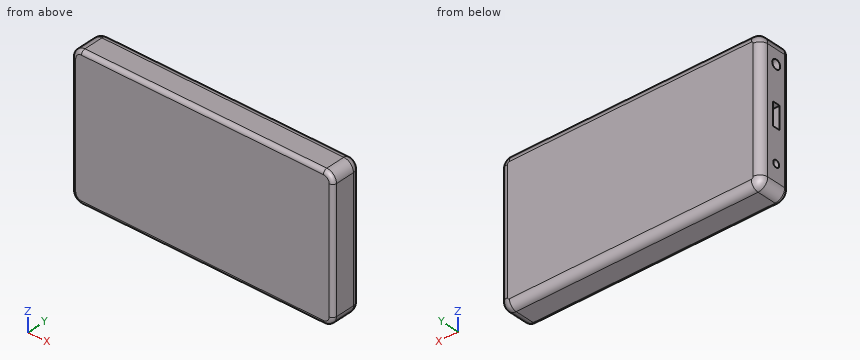
```python
from build123d import *

# Parameters (mm, degrees)
SKETCH1_W           = 270
SKETCH1_H           = 145
BOSS_EXTRUDE1_DEPTH = 32
FILLET1_R           = 8
FILLET2_R           = 10
FILLET3_R           = 4
SKETCH2_R           = 3.521962556
SKETCH2_R_2         = 4.707421484
SKETCH2_W           = 23.153777818
SKETCH2_H           = 8.080231906
CUT_EXTRUDE1_DEPTH  = 33


with BuildPart() as part:
    # Sketch1 → Boss-Extrude1 (new body)
    with BuildSketch(Plane(origin=(0, 0, 0), x_dir=(1, 0, 0), z_dir=(0, 1, 0))):
        Rectangle(SKETCH1_W, SKETCH1_H)
    extrude(amount=BOSS_EXTRUDE1_DEPTH)

    # Fillet1
    fillet1_edges = [part.edges().sort_by_distance(p)[0] for p in [
        (-135, 32, 0),
        (0, 32, 72.5),
        (135, 32, 0),
        (0, 32, -72.5),
    ]]
    fillet(fillet1_edges, radius=FILLET1_R)

    # Fillet2
    # the kernel refuses this fillet: 10 mm, written as the material it takes off along each edge
    with BuildSketch(Plane(origin=(-125, 32, 62.5), x_dir=(-1, 0, 0), z_dir=(0, 0, -1))) as fillet2_piece_1:
        with BuildLine():
            CenterArc((2, -8), 8, 0, 90)
            Line((10, -8), (10, 0))
            Line((10, 0), (2, 0))
        make_face()
    revolve(axis=Axis((-125, 32, 62.5), (0, 1, 0)), revolution_arc=90, mode=Mode.SUBTRACT)
    with BuildSketch(Plane(origin=(-125, 32, -62.5), x_dir=(0, 0, -1), z_dir=(1, 0, 0))) as fillet2_piece_2:
        with BuildLine():
            CenterArc((2, -8), 8, 0, 90)
            Line((10, -8), (10, 0))
            Line((10, 0), (2, 0))
        make_face()
    revolve(axis=Axis((-125, 32, -62.5), (0, 1, 0)), revolution_arc=90, mode=Mode.SUBTRACT)
    with BuildSketch(Plane(origin=(125, 32, 62.5), x_dir=(0, 0, 1), z_dir=(-1, 0, 0))) as fillet2_piece_3:
        with BuildLine():
            CenterArc((2, -8), 8, 0, 90)
            Line((10, -8), (10, 0))
            Line((10, 0), (2, 0))
        make_face()
    revolve(axis=Axis((125, 32, 62.5), (0, 1, 0)), revolution_arc=90, mode=Mode.SUBTRACT)
    with BuildSketch(Plane(origin=(125, 32, -62.5), x_dir=(1, 0, 0), z_dir=(0, 0, 1))) as fillet2_piece_4:
        with BuildLine():
            CenterArc((2, -8), 8, 0, 90)
            Line((10, -8), (10, 0))
            Line((10, 0), (2, 0))
        make_face()
    revolve(axis=Axis((125, 32, -62.5), (0, 1, 0)), revolution_arc=90, mode=Mode.SUBTRACT)
    with BuildSketch(Plane(origin=(135, -25, -72.5), x_dir=(-1, 0, 0), z_dir=(0, 1, 0)), Plane(origin=(135, -25, 72.5), x_dir=(0, 0, -1), z_dir=(0, 1, 0))) as fillet2_piece_5:
        with BuildLine():
            CenterArc((FILLET2_R, FILLET2_R), FILLET2_R, 180, 90)
            Line((0, FILLET2_R), (0, 0))
            Line((0, 0), (FILLET2_R, 0))
        make_face()
    extrude(amount=57, mode=Mode.SUBTRACT)
    with BuildSketch(Plane(origin=(-135, -25, -72.5), x_dir=(1, 0, 0), z_dir=(0, 1, 0)), Plane(origin=(-135, -25, 72.5), x_dir=(0, 0, -1), z_dir=(0, 1, 0))) as fillet2_piece_6:
        with BuildLine():
            CenterArc((FILLET2_R, -FILLET2_R), FILLET2_R, 90, 90)
            Line((0, -FILLET2_R), (0, 0))
            Line((0, 0), (FILLET2_R, 0))
        make_face()
    extrude(amount=57, mode=Mode.SUBTRACT)

    # Fillet3
    fillet3_edges = [part.edges().sort_by_distance(p)[0] for p in [
        (-135, 0, 0),
        (135, 0, 0),
        (0, 0, 72.5),
        (0, 0, -72.5),
        (132.071067812, 0, 69.571067812),
        (132.071067812, 0, -69.571067812),
        (-132.071067812, 0, 69.571067812),
        (-132.071067812, 0, -69.571067812),
    ]]
    fillet(fillet3_edges, radius=FILLET3_R)

    # Sketch2 → Cut-Extrude1 (cut)
    with BuildSketch(Plane.ZY.offset(135)):
        with Locations((-45.200201046, 14)):
            Circle(SKETCH2_R)
        with Locations((48.220259023, 14)):
            Circle(SKETCH2_R_2)
        with Locations((0, 14)):
            Rectangle(SKETCH2_W, SKETCH2_H)
    extrude(amount=-CUT_EXTRUDE1_DEPTH, mode=Mode.SUBTRACT)


solid = part.part
```
Here's how the part is built. I have some questions about the finished solid (model axes, mm). Coordinates: 2 decimals unless noted, no trailing zeros. Order: outer loops, then holes, each group sorted by start corner. A loop starts at its lowest first (then second) coordinate and runs counter-clockwise, first axis right, second up. Notation, with made-up numbers: (59, 24.5) - (103, 24.5) arc R19 ccw to (103, 46.5) - close; hole circle Ø8 at (54.5, 10). An arc over 180 degrees is marked (long way). One line per question, with ' | ' between items. Start each with the question number.
1. If we section it at A-A (y = 14): Write out the boundary of the cut face in (x, z), and give its area (3 significant figures).
2. Please list where these lines run through material, in increasing order: line 1 along Z through (x, y) = (-116, 13); line 2 along X through (y, z) = (25, 8); line 3 along X through (y, z) = (24.5, -44). Write a range as [from, to].
3. I'm going to push a flat-ended pin straight in: pin 1 Ø3.5 at (y, z) = (15, -45.5) entering from -X. Where does the tip first touch, or does it pass through?
Model answer:
1) outline: (-135, -62.5) arc R10 ccw to (-125, -72.5) - (125, -72.5) arc R10 ccw to (135, -62.5) - (135, 62.5) arc R10 ccw to (125, 72.5) - (-125, 72.5) arc R10 ccw to (-135, 62.5) - (-135, 52.93) - (-102, 52.93) - (-102, 43.51) - (-135, 43.51) - (-135, 11.58) - (-102, 11.58) - (-102, -11.58) - (-135, -11.58) - (-135, -41.68) - (-102, -41.68) - (-102, -48.72) - (-135, -48.72) - close | area: 37,800 mm²
2) line 1: z = [-72.5, -48.58], [-41.82, -11.58], [11.58, 43.62], [52.82, 72.5] | line 2: x = [-134.94, 134.94] | line 3: x = [-134.98, 134.98]
3) pin 1: stops at x = -102
